```python
from build123d import *

# Parameters (mm, degrees)
SKETCH1_W           = 38.1
SKETCH1_H           = 53.975
BOSS_EXTRUDE1_DEPTH = 3.175
SKETCH2_W           = 38.1
SKETCH2_H           = 53.975
SKETCH2_W_2         = 31.75
SKETCH2_H_2         = 47.625
BOSS_EXTRUDE2_DEPTH = 90.4875
CHAMFER1_SIZE       = 3.81


with BuildPart() as part:
    # Sketch1 → Boss-Extrude1 (new body)
    with BuildSketch(Plane(origin=(0, 0, 0), x_dir=(1, 0, 0), z_dir=(0, 1, 0))):
        with Locations((-33.545007613, -37.607739585)):
            Rectangle(SKETCH1_W, SKETCH1_H)
    extrude(amount=BOSS_EXTRUDE1_DEPTH)

    # Sketch2 → Boss-Extrude2 (add)
    with BuildSketch(Plane(origin=(0, 3.175, 0), x_dir=(1, 0, 0), z_dir=(0, 1, 0))):
        with Locations((-33.545007613, -37.607739585)):
            Rectangle(SKETCH2_W, SKETCH2_H)
        with Locations((-33.545007613, -37.607739585)):
            Rectangle(SKETCH2_W_2, SKETCH2_H_2, mode=Mode.SUBTRACT)
    extrude(amount=BOSS_EXTRUDE2_DEPTH)

    # Chamfer1
    chamfer1_edges = [part.edges().sort_by_distance(p)[0] for p in [
        (-52.595007613, 46.83125, 10.620239585),
        (-14.495007613, 46.83125, 10.620239585),
        (-14.495007613, 46.83125, 64.595239585),
        (-52.595007613, 46.83125, 64.595239585),
    ]]
    chamfer(chamfer1_edges, length=CHAMFER1_SIZE)


solid = part.part
```
CAD build for the part. Positions are in the model's coordinates, mm. A direction names the side the tool comes from. Coordinates: 2 decimals unless noted, no trailing zeros. Order: outer loops, then holes, each group sorted by start corner. A loop starts at its lowest first (then second) coordinate and runs counter-clockwise, first axis right, second up. Notation, with made-up numbers: (69.25, 41.5) - (99.25, 41.5) arc R22 ccw to (99.25, 55.5) - close; hole circle Ø2 at (-32, 46.5). An arc over 180 degrees is marked (long way). Use a Markdown table: item, result. Add a question column.
(1) Pull direction Z, two halves, no side cores. Call faces 3 (the face through (-16.37, 46.18, 62.66)), 4 (the face through (-14.495, 46, 38)), 5 (the face through (-34, 3.175, 37)), 6 (the face through (-16.427, 47.487, 12.499)): +Z half, -Z half, draft (parallel to the pull), parting line (faces both ways), or undercut.
(2) Saw through at C-C (x = -36). Give the cut face in (y, z) (1 decimal).
(3) Which spindle directions (+Z, -Z, +X, -X, +Y, -Y) get a long thin tool onto all of the face, cutting with end or side? Do faces 1 (the face through (-34, 0, 37)), 2 (the face through (-17.67, 48, 38)). Say none if no direction does.
(4) Flat gauge pin, fed straight in: pin 1 (6 mm diameter, centred on x = -44.5, z = 54, fed in from +Y) (3 decimals). Where does the tip first touch, or does it go through?
(5) Drill centre lines: line 1 along X through (y, z) = (69.5, 58.5) (3 decimals); line 2 along Z through (x, y) = (-37, 58.5); line 3 along Y through (x, z) = (-31.5, 16) (3 decimals). Where is each one in solid material? Low to high. Write a range as [from, to].
(6) Saw through at A-A (y = 55). Give the cut face in (x, z) (3 decimals).
(7) Saw through at B-B (z = 33.5). Give the cut face in (x, y) (1 decimal).
Solved:
| question | item | result |
|---|---|---|
| 1 | face 3 | +Z half |
| 1 | face 4 | draft |
| 1 | face 5 | undercut |
| 1 | face 6 | -Z half |
| 2 | outline | (0, 10.6) - (93.7, 10.6) - (93.7, 13.8) - (3.2, 13.8) - (3.2, 61.4) - (93.7, 61.4) - (93.7, 64.6) - (0, 64.6) - close |
| 3 | face 1 | +Z, -Z, +X, -X, -Y |
| 3 | face 2 | +Y |
| 4 | pin 1 | stops at y = 3.175 |
| 5 | line 1 | x = [-52.595, -49.42], [-17.67, -14.495] |
| 5 | line 2 | z = [10.62, 13.8], [61.42, 64.6] |
| 5 | line 3 | y = [0, 3.175] |
| 6 | outline | (-52.595, 14.43) - (-48.785, 10.62) - (-18.305, 10.62) - (-14.495, 14.43) - (-14.495, 60.785) - (-18.305, 64.595) - (-48.785, 64.595) - (-52.595, 60.785) - close; hole (-49.42, 13.795) - (-17.67, 13.795) - (-17.67, 61.42) - (-49.42, 61.42) - close |
| 7 | outline | (-52.6, 0) - (-14.5, 0) - (-14.5, 93.7) - (-17.7, 93.7) - (-17.7, 3.2) - (-49.4, 3.2) - (-49.4, 93.7) - (-52.6, 93.7) - close |
